Verification items for the finished model (mm, model axes). Coordinates: 2 decimals unless noted, no trailing zeros. Order: outer loops, then holes, each group sorted by start corner. A loop starts at its lowest first (then second) coordinate and runs counter-clockwise, first axis right, second up. Notation, with made-up numbers: (21, 81.5) -> (78, 81.5) arc R21 ccw to (78, 111.5) -> close; hole circle Ø5 at (53.25, 89). An arc over 180 degrees is marked (long way). Answer as CSV lines item,"result".
```python
from build123d import *

# Parameters (mm, degrees)
SKETCH1_W           = 300
SKETCH1_H           = 150
SKETCH1_R           = 14.235
BOSS_EXTRUDE1_DEPTH = 3
CUT_EXTRUDE1_REACH  = 5
SKETCH2_R           = 3.225
SKETCH3_R           = 2.4892
CUT_EXTRUDE2_DEPTH  = 4


with BuildPart() as part:
    # Sketch1 → Boss-Extrude1 (new body)
    with BuildSketch(Plane(origin=(0, 0, 0), x_dir=(0, 0, -1), z_dir=(1, 0, 0))):
        with Locations((150, 75)):
            Rectangle(SKETCH1_W, SKETCH1_H)
        with Locations((30, 55)):
            Circle(SKETCH1_R, mode=Mode.SUBTRACT)
    extrude(amount=BOSS_EXTRUDE1_DEPTH)

    # Sketch2 → Cut-Extrude1 (cut, up to next)
    with BuildSketch(Plane.ZY, mode=Mode.PRIVATE) as cut_extrude1_sk1:
        with Locations((-290, 140)):
            Circle(SKETCH2_R)
    cut_extrude1_tool1 = extrude(cut_extrude1_sk1.sketch, amount=-CUT_EXTRUDE1_REACH, mode=Mode.PRIVATE) & part.part
    add(cut_extrude1_tool1.solids().sort_by_distance((0, 140, -290))[0], mode=Mode.SUBTRACT)
    # Sketch2 → Cut-Extrude1 (cut, up to next)
    with BuildSketch(Plane.ZY, mode=Mode.PRIVATE) as cut_extrude1_sk2:
        with Locations((-10, 110)):
            Circle(SKETCH2_R)
    cut_extrude1_tool2 = extrude(cut_extrude1_sk2.sketch, amount=-CUT_EXTRUDE1_REACH, mode=Mode.PRIVATE) & part.part
    add(cut_extrude1_tool2.solids().sort_by_distance((0, 110, -10))[0], mode=Mode.SUBTRACT)
    # Sketch2 → Cut-Extrude1 (cut, up to next)
    with BuildSketch(Plane.ZY, mode=Mode.PRIVATE) as cut_extrude1_sk3:
        with Locations((-290, 30)):
            Circle(SKETCH2_R)
    cut_extrude1_tool3 = extrude(cut_extrude1_sk3.sketch, amount=-CUT_EXTRUDE1_REACH, mode=Mode.PRIVATE) & part.part
    add(cut_extrude1_tool3.solids().sort_by_distance((0, 30, -290))[0], mode=Mode.SUBTRACT)
    # Sketch2 → Cut-Extrude1 (cut, up to next)
    with BuildSketch(Plane.ZY, mode=Mode.PRIVATE) as cut_extrude1_sk4:
        with BuildLine():
            Line((-246.901029004, 58.225), (-206.901029004, 58.225))
            ThreePointArc((-206.901029004, 58.225), (-203.676029004, 55), (-206.901029004, 51.775))
            Line((-206.901029004, 51.775), (-246.901029004, 51.775))
            ThreePointArc((-246.901029004, 51.775), (-250.126029004, 55), (-246.901029004, 58.225))
        make_face()
    cut_extrude1_tool4 = extrude(cut_extrude1_sk4.sketch, amount=-CUT_EXTRUDE1_REACH, mode=Mode.PRIVATE) & part.part
    add(cut_extrude1_tool4.solids().sort_by_distance((0, 55, -226.901029))[0], mode=Mode.SUBTRACT)
    # Sketch2 → Cut-Extrude1 (cut, up to next)
    with BuildSketch(Plane.ZY, mode=Mode.PRIVATE) as cut_extrude1_sk5:
        with BuildLine():
            Line((-206.901029004, 111.77), (-246.901029004, 111.77))
            ThreePointArc((-246.901029004, 111.77), (-250.131029004, 115), (-246.901029004, 118.23))
            Line((-246.901029004, 118.23), (-206.901029004, 118.23))
            ThreePointArc((-206.901029004, 118.23), (-203.671029004, 115), (-206.901029004, 111.77))
        make_face()
    cut_extrude1_tool5 = extrude(cut_extrude1_sk5.sketch, amount=-CUT_EXTRUDE1_REACH, mode=Mode.PRIVATE) & part.part
    add(cut_extrude1_tool5.solids().sort_by_distance((0, 115, -226.901029))[0], mode=Mode.SUBTRACT)
    # Sketch2 → Cut-Extrude1 (cut, up to next)
    with BuildSketch(Plane.ZY, mode=Mode.PRIVATE) as cut_extrude1_sk6:
        with BuildLine():
            Line((-246.901029004, 41.775), (-206.901029004, 41.775))
            ThreePointArc((-206.901029004, 41.775), (-203.676029004, 38.55), (-206.901029004, 35.325))
            Line((-206.901029004, 35.325), (-246.901029004, 35.325))
            ThreePointArc((-246.901029004, 35.325), (-250.126029004, 38.55), (-246.901029004, 41.775))
        make_face()
    cut_extrude1_tool6 = extrude(cut_extrude1_sk6.sketch, amount=-CUT_EXTRUDE1_REACH, mode=Mode.PRIVATE) & part.part
    add(cut_extrude1_tool6.solids().sort_by_distance((0, 38.55, -226.901029))[0], mode=Mode.SUBTRACT)
    # Sketch2 → Cut-Extrude1 (cut, up to next)
    with BuildSketch(Plane.ZY, mode=Mode.PRIVATE) as cut_extrude1_sk7:
        with BuildLine():
            Line((-246.901029004, 13.775), (-206.901029004, 13.775))
            ThreePointArc((-206.901029004, 13.775), (-203.676029004, 10.55), (-206.901029004, 7.325))
            Line((-206.901029004, 7.325), (-246.901029004, 7.325))
            ThreePointArc((-246.901029004, 7.325), (-250.126029004, 10.55), (-246.901029004, 13.775))
        make_face()
    cut_extrude1_tool7 = extrude(cut_extrude1_sk7.sketch, amount=-CUT_EXTRUDE1_REACH, mode=Mode.PRIVATE) & part.part
    add(cut_extrude1_tool7.solids().sort_by_distance((0, 10.55, -226.901029))[0], mode=Mode.SUBTRACT)

    # Sketch3 → Cut-Extrude2 (cut, through all)
    with BuildSketch(Plane(origin=(3, 0, 0), x_dir=(0, 0, -1), z_dir=(1, 0, 0))):
        with Locations((14.005743185, 74.73179538)):
            Circle(SKETCH3_R)
        with Locations((45.994256815, 35.26820462)):
            Circle(SKETCH3_R)
    extrude(amount=-CUT_EXTRUDE2_DEPTH, mode=Mode.SUBTRACT)


solid = part.part
```
Item 1: Section check C-C, the plane y = 55. Record the boundary of the cut face in (x, z) (3 decimals).
Answer list:
outline,"(0, -300) -> (3, -300) -> (3, -250.126) -> (0, -250.126) -> close; (0, -203.676) -> (3, -203.676) -> (3, -44.235) -> (0, -44.235) -> close; (0, -15.765) -> (3, -15.765) -> (3, 0) -> (0, 0) -> close"
Item 2: Thickness scan on line 1 (Y direction, x = 1.2, z = -215.5) (3 decimals); line 2 (Z direction, x = 2.1, y = 10); line 3 (Y direction, x = 2.35, z = -30) (3 decimals). Record the ranges inside material, lowest first.
Answer list:
line 1,"0 to 7.325, 13.775 to 35.325, 41.775 to 51.775, 58.225 to 111.77, 118.23 to 150"
line 2,"-300 to -250.08, -203.72 to 0"
line 3,"0 to 40.765, 69.235 to 150"
Item 3: Section check A-A, the plane z = -290. Record the boundary of the cut face in (x, y) (3 decimals), plus the area to 3 significant figures.
Answer list:
outline,"(0, 0) -> (3, 0) -> (3, 26.775) -> (0, 26.775) -> close; (0, 33.225) -> (3, 33.225) -> (3, 136.775) -> (0, 136.775) -> close; (0, 143.225) -> (3, 143.225) -> (3, 150) -> (0, 150) -> close"
area,"411 mm2"
Item 4: Section check B-B, the plane z = -30. Record the boundary of the cut face in (x, y) (3 decimals).
Answer list:
outline,"(0, 0) -> (3, 0) -> (3, 40.765) -> (0, 40.765) -> close; (0, 69.235) -> (3, 69.235) -> (3, 150) -> (0, 150) -> close"
Item 5: Depth check by flat-ended pin: pin 1 Ø1.5 at (x, z) = (1.5, -222.5) entering from -Y. Enter the tip coordinate at first touch or a pass-through.
Answer list:
pin 1,"y = 0"
Item 6: Release check for a two-part mould opening along Z. For faces 1 (the flat face through (0, 76, -148)), 2 (the cylindrical face through (1.48, 106.85, -10.7)) record: +Z half, -Z half, draft (parallel to the pull), parting line (faces both ways), or undercut.
Answer list:
face 1,"draft"
face 2,"undercut"
Item 7: Section check D-D, the plane y = 140. Record the boundary of the cut face in (x, z) (3 decimals).
Answer list:
outline,"(0, -300) -> (3, -300) -> (3, -293.225) -> (0, -293.225) -> close; (0, -286.775) -> (3, -286.775) -> (3, 0) -> (0, 0) -> close"
